```python
from build123d import *

# Parameters (mm, degrees)
SKETCH1_R                = 1.6
SKETCH1_R_2              = 3
BOSS_EXTRUDE1_DEPTH      = 4
BOSS_EXTRUDE2_DEPTH      = 5
BOSS_EXTRUDE2_DEPTH_BACK = 9
CHAMFER1_SIZE            = 5


with BuildPart() as part:
    # Sketch1 → Boss-Extrude1 (new body)
    with BuildSketch(Plane(origin=(0, 0, 0), x_dir=(0, 0, -1), z_dir=(1, 0, 0))):
        with BuildLine():
            Line((0.053412883, 6.49978054), (75, 5.883896162))
            ThreePointArc((75, 5.883896162), (77.997285796, 3.011480877), (75.25493857, -0.105251932))
            Line((75.25493857, -0.105251932), (27, -4.220820858))
            Line((27, -4.220820858), (27, -12))
            ThreePointArc((27, -12), (22, -17), (17, -12))
            Line((17, -12), (17, -5.073701216))
            Line((17, -5.073701216), (0.552366901, -6.476487536))
            ThreePointArc((0.552366901, -6.476487536), (-6.495200196, -0.249748712), (0.053412883, 6.49978054))
        make_face()
        with Locations((22, -12)):
            Circle(SKETCH1_R, mode=Mode.SUBTRACT)
        Circle(SKETCH1_R_2, mode=Mode.SUBTRACT)
    extrude(amount=BOSS_EXTRUDE1_DEPTH)

    # Sketch2 → Boss-Extrude2 (add, two sides: drawn at the far end of the back side and taken through both)
    with BuildSketch(Plane(origin=(4, 0, 0), x_dir=(0, 0, -1), z_dir=(1, 0, 0)).offset(-BOSS_EXTRUDE2_DEPTH_BACK)):
        with BuildLine():
            Line((70.003692287, 2.691778393), (70.128057116, -0.54251358))
            Line((70.128057116, -0.54251358), (75.25493857, -0.105251932))
            ThreePointArc((75.25493857, -0.105251932), (77.997285796, 3.011480877), (75, 5.883896162))
            Line((75, 5.883896162), (69.879331086, 5.925975997))
            Line((69.879331086, 5.925975997), (70.003692287, 2.691778393))
        make_face()
    extrude(amount=BOSS_EXTRUDE2_DEPTH + BOSS_EXTRUDE2_DEPTH_BACK)

    # Chamfer1
    chamfer1_edges = [part.edges().sort_by_distance(p)[0] for p in [
        (0, 2.691731208, -70.003694101),
        (4, 2.691731208, -70.003694101),
    ]]
    chamfer(chamfer1_edges, length=CHAMFER1_SIZE - 0.0001)  # a hair under: the kernel refuses the full size


solid = part.part
```
Geometry check sheet. Reference: the model listing, model coordinates, mm. A direction names the side the tool comes from. Coordinates: 2 decimals unless noted, no trailing zeros. Order: outer loops, then holes, each group sorted by start corner. A loop starts at its lowest first (then second) coordinate and runs counter-clockwise, first axis right, second up. Notation, with made-up numbers: M -28,55 L -3,55 A18 cw -3,62 Z; hole C 9,-20 d5. An arc over 180 degrees is marked long. Answer as a JSON object with one key per item and string values.
Q1. Depth check by flat-ended pin: pin 1 Ø3 at (y, z) = (2, -60) entering from -X; pin 2 Ø1.2 at (x, y) = (2, -10) entering from -Z; pin 3 Ø6 at (x, z) = (2.5, -32) entering from -Y. Enter the tip coordinate at first touch or a pass-through.
Results are:
{"pin 1": "stops at x = 0", "pin 2": "stops at z = -27", "pin 3": "stops at y = -4.05"}
Q2. Cross-section at A-A on x = 3.25. Record the cut outline in (y, z), and give its area (3 significant figures).
Results are:
{"outline": "M -12,-27 L -4.22,-27 L -0.11,-75.25 A3 ccw 5.88,-75 L 6.5,-0.05 A6.5 ccw long -6.48,-0.55 L -5.07,-17 L -12,-17 A5 ccw Z; hole C -12,-22 d3.2; hole C 0,0 d6", "area": "871 mm²"}
Q3. Cross-section at D-D on x = -1.5. Record the cut outline in (y, z).
Results are:
{"outline": "M -0.84,-66.64 L -0.11,-75.25 A3 ccw 5.88,-75 L 5.95,-66.38 Z"}
Q4. Release check for a two-part mould opening along Y. For faces 5 (the cylindrical face through (1.9, 2.9, -78)), 6 (the cylindrical face through (1.97, -13.42, -22.74)), 7 (the flat face through (0, 0, -30)) record: released by +Y, released by -Y, zero draft, split by the parting line, or undercut.
Results are:
{"face 5": "split by the parting line", "face 6": "undercut", "face 7": "zero draft"}
Q5. Tool access check on faces 1 (the flat face through (4, 0, -30)), 2 (the flat face through (2, -8, -27)), 3 (the flat face through (2, -9, -17)), 4 (the flat face through (-5, 3, -74)). Record the directions out of +Z, -Z, +X, -X, +Y, -Y that give a thin tool (end or side, any length) a straight path to the whole face; none if there is none.
Results are:
{"face 1": "+Z, +X, +Y, -Y", "face 2": "-Z, +X, -X, -Y", "face 3": "+X, -X, -Y", "face 4": "+Z, -Z, -X, +Y, -Y"}
Q6. Cross-section at C-C on z = -71.5. Record the cut outline in (x, y), and give its area (3 significant figures).
Results are:
{"outline": "M -5,-0.43 L 9,-0.43 L 9,5.91 L -5,5.91 Z", "area": "88.7 mm²"}
Q7. Cross-section at B-B on z = -22. Record the cut outline in (x, y), and give its area (3 significant figures).
Results are:
{"outline": "M 0,-17 L 4,-17 L 4,-13.6 L 0,-13.6 Z; M 0,-10.4 L 4,-10.4 L 4,6.32 L 0,6.32 Z", "area": "80.5 mm²"}
Q8. Scan lines: line 1 (Y direction, x = 1.55, z = 0); line 2 (X direction, y = 3, z = -65); line 3 (Y direction, x = 2.6, z = -22). Record each from-to range of solid material in increasing order.
Results are:
{"line 1": "y = -6.5 to -3, 3 to 6.5", "line 2": "x = -0.01 to 4.01", "line 3": "y = -17 to -13.6, -10.4 to 6.32"}
